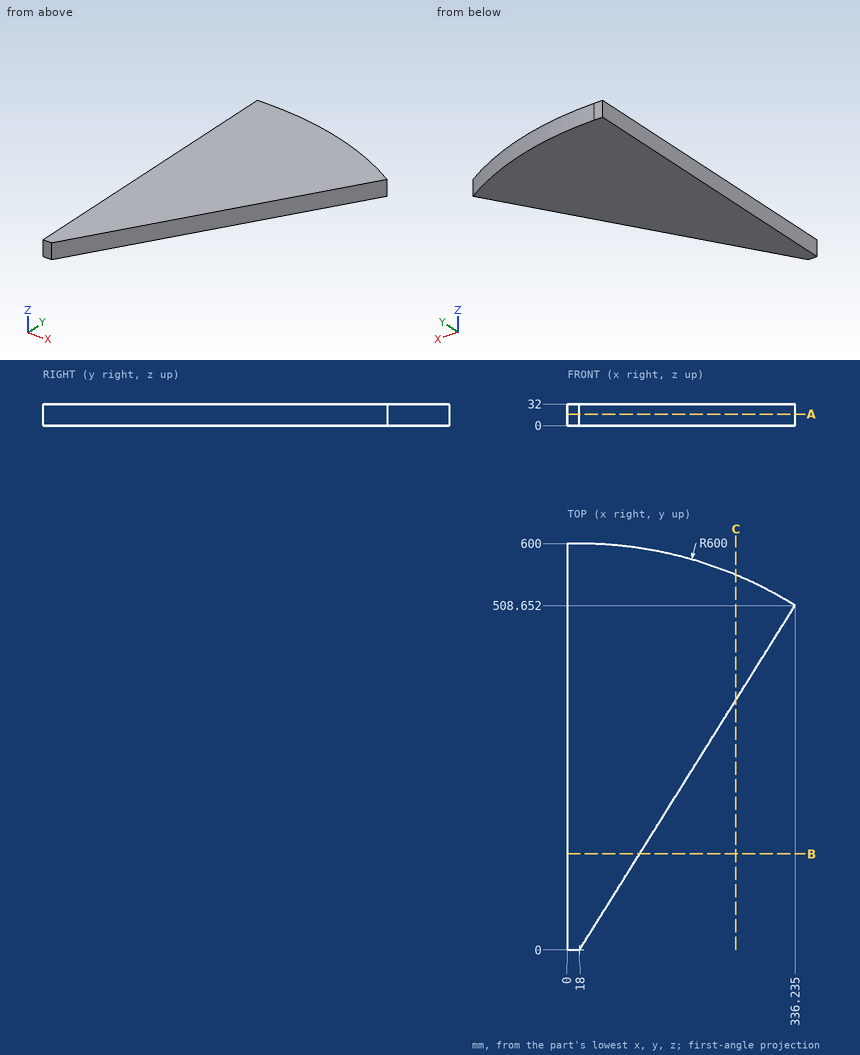
Could you check a few things on this drawing? It's one solid part, dimensions in mm from its lowest x, y, z. Round coordinates to 2 decimals unless told otherwise and drop trailing zeros. Loops run counter-clockwise (first coordinate to the right, second up) from the corner with the lowest first, then second, coordinate; pieces in that order, holes last.
Q1. I want a section at A-A (z = 17). Write out the boundary of the cut face in (x, y) (1 decimal), and give its area (3 significant figures).
Q2. For P1, Ø4, axis at y = 69.5, z = 9.5, coming from the +X side; P2, Ø8, axis at x = 155.5, z = 15, coming from the -Y side, each with a flat end and sliding along its axis, tell me the tip position at first contact or that it passes through.
Q3. Please list where these lines run through material, in increasing order: L1, parallel to Y at x = 256.5, z = 1 (1 decimal); L2, parallel to X at y = 317, z = 30; L3, parallel to Y at x = 126, z = 25.
Q4. I want a section at C-C (x = 249). Write out the boundary of the cut face in (y, z).
Q5. I want a section at B-B (y = 142). Write out the boundary of the cut face in (x, z).
Answer below:
1. outline: (0, 0) - (18, 0) - (336.2, 508.7) arc R600 ccw to (18, 600) - (0, 600) - close
1. area: 111,000 mm2
2. P1: stops at x = 62.73
2. P2: stops at y = 213.38
3. L1: y = 381.2 to 550.6
3. L2: x = 0 to 216.33
3. L3: y = 172.62 to 590.2
4. outline: (369.22, 0) - (553.75, 0) - (553.75, 32) - (369.22, 32) - close
5. outline: (0, 0) - (106.84, 0) - (106.84, 32) - (0, 32) - close
